Can you work these out from the model? Positions are in its coordinate system, mm. A direction names the side the tool comes from. Give positions to 0.01 mm unless a question says otherwise; leave off trailing zeros. Loops run counter-clockwise (first coordinate to the right, second up) from the corner with the lowest first, then second, coordinate; pieces in that order, holes last. Notation, with made-up numbers: (-25, 22.25) -> (-8, 22.25) arc R17 cw to (-8, 47.25) -> close; hole circle Ø1 at (15.25, -19.5). An arc over 180 degrees is marked (long way). Return JSON: item names as keys, results as strings. Group by question number.
Q1. Will these pins go through, and if not, where does the flat tip stop? pin 1 (1.5 mm diameter, centred on x = 3, z = 1.5, fed in from +Y); pin 2 (1.5 mm diameter, centred on x = 2.5, y = 17.5, fed in from +Z).
Q2. Which directions (+Z, -Z, +X, -X, +Y, -Y) give clear straight access to the entire face, cutting with the end or side of a thin tool? Please do faces 1 (the flat face through (0, 0, 0)), 2 (the cylindrical face through (-0.321, 27.062, 2.443)).
Q3. Suppose I cut it at C-C, the plane y = 5. Please give me the cut outline in (x, z).
Q4. I need wall thicknesses on line 1 along X through (y, z) = (16.5, 2); line 2 along Y through (x, z) = (1.75, -2); line 3 along Z through (x, y) = (-2, 9.5). Which ranges of each line are inside material? Lowest first, please. Write a range as [from, to].
Q5. Suppose I cut it at A-A, the plane x = 0. Please give me the cut outline in (y, z).
Q6. Suppose I cut it at B-B, the plane z = 0. Please give me the cut outline in (x, y), and give its area (3 significant figures).
Autodesk Inventor part; units mm, degrees
ref_plane "YZ Plane" through (0, 0, 0) normal (1, 0, 0) x (0, 1, 0)
ref_plane "XZ Plane" through (0, 0, 0) normal (0, 1, 0) x (-1, 0, 0)
ref_plane "XY Plane" through (0, 0, 0) normal (0, 0, 1) x (1, 0, 0)
sketch "Sketch1" plane through (0, 0, 0) normal (0, 1, 0) x (-1, 0, 0)
  circle A0 centre (0, 0) radius 4
  dimension "d0" = 8
extrude "Extrusion1" add sketch "Sketch1" along normal blind 16
chamfer "Chamfer1" distance 1.5 angle 45 1 edges at (4, 16, 0)
sketch "Sketch2" plane through (0, 16, 0) normal (0, 1, 0) x (1, 0, 0)
  circle A0 centre (0, 0) radius 2.5
extrude "Extrusion2" add sketch "Sketch2" along normal blind 10
chamfer "Chamfer2" distance 0.3 distance2 1 1 edges at (-2.5, 26, 0) measured on face at (1.2612, 26, 0.6619)
sketch "Sketch3" plane through (0, 26, 0) normal (0, 1, 0) x (1, 0, 0)
  circle A0 centre (0, 0) radius 2.5
  circle A1 centre (0, 0) radius 2.4644
extrude "Extrusion3" add sketch "Sketch3" along normal blind 2 contours A1
chamfer "Chamfer3" distance 0.15 angle 45 1 edges at (-2.4644, 26, 0)
properties part number "McCrea_wrist_Walle"
Ans:
{
 "1": {"pin 1": "stops at y = 15.9", "pin 2": "stops at z = 1.79"},
 "2": {"face 1": "+Z, -Z, +X, -X, -Y", "face 2": "+Y"},
 "3": {"outline": "circle Ø8 at (0, 0)"},
 "4": {"line 1": "x = [-1.5, 1.5]", "line 2": "y = [0, 15.84]", "line 3": "z = [-3.46, 3.46]"},
 "5": {"outline": "(0, -4) -> (14.5, -4) -> (16, -2.5) -> (25, -2.5) -> (26, -2.2) -> (26, -2.31) -> (26.15, -2.46) -> (28, -2.46) -> (28, 2.46) -> (26.15, 2.46) -> (26, 2.31) -> (26, 2.2) -> (25, 2.5) -> (16, 2.5) -> (14.5, 4) -> (0, 4) -> close"},
 "6": {"outline": "(-4, 0) -> (4, 0) -> (4, 14.5) -> (2.5, 16) -> (2.5, 25) -> (2.2, 26) -> (2.31, 26) -> (2.46, 26.15) -> (2.46, 28) -> (-2.46, 28) -> (-2.46, 26.15) -> (-2.31, 26) -> (-2.2, 26) -> (-2.5, 25) -> (-2.5, 16) -> (-4, 14.5) -> close", "area": "185 mm^2"}
}
